Can you work these out from the model? Positions are in its coordinate system, mm. Coordinates: 2 decimals unless noted, no trailing zeros. Write item = value, one per line.
```python
from build123d import *

# Parameters (mm, degrees)
F1_DEPTH = 504


with BuildPart() as f1:
    # F0 (on Top) → F1 (new body)
    with BuildSketch(Plane.XY):
        Polygon((12, 4), (-12, 4), (-12, -4), (-1.9, -4), (-1.9, 2.8), (1.9, 2.8), (1.9, -4), (12, -4), align=None)
        with BuildLine():
            Line((-9.623275, -3.2), (-11.2, -3.2))
            Line((-11.2, -3.2), (-11.2, 3.2))
            Line((-11.2, 3.2), (-9.623275, 3.2))
            ThreePointArc((-9.623275, 3.2), (-9.422747, 2.985045), (-9.502111, 2.701993))
            Line((-9.502111, 2.701993), (-10.097086, 2.107018))
            ThreePointArc((-10.097086, 2.107018), (-10.312788, 1.783105), (-10.388512, 1.401382))
            Line((-10.388512, 1.401382), (-10.388512, 1.218503))
            ThreePointArc((-10.388512, 1.218503), (-10.25826, 1.031059), (-10.03716, 1.087764))
            ThreePointArc((-10.03716, 1.087764), (-8.786443, 1.659163), (-7.537162, 1.084629))
            ThreePointArc((-7.537162, 1.084629), (-7.316853, 1.031709), (-7.188512, 1.218431))
            Line((-7.188512, 1.218431), (-7.188512, 1.397588))
            ThreePointArc((-7.188512, 1.397588), (-7.264631, 1.780269), (-7.481401, 2.104691))
            Line((-7.481401, 2.104691), (-8.076376, 2.699666))
            ThreePointArc((-8.076376, 2.699666), (-8.154767, 2.986603), (-7.947546, 3.2))
            Line((-7.947546, 3.2), (-2.8, 3.2))
            Line((-2.8, 3.2), (-2.8, -3.2))
            Line((-2.8, -3.2), (-7.947546, -3.2))
            ThreePointArc((-7.947546, -3.2), (-8.154767, -2.986603), (-8.076376, -2.699666))
            Line((-8.076376, -2.699666), (-7.481401, -2.104691))
            ThreePointArc((-7.481401, -2.104691), (-7.264631, -1.780269), (-7.188512, -1.397588))
            Line((-7.188512, -1.397588), (-7.188512, -1.218431))
            ThreePointArc((-7.188512, -1.218431), (-7.316853, -1.031709), (-7.537162, -1.084629))
            ThreePointArc((-7.537162, -1.084629), (-8.786443, -1.659163), (-10.03716, -1.087764))
            ThreePointArc((-10.03716, -1.087764), (-10.25826, -1.031059), (-10.388512, -1.218503))
            Line((-10.388512, -1.218503), (-10.388512, -1.401382))
            ThreePointArc((-10.388512, -1.401382), (-10.312788, -1.783105), (-10.097086, -2.107018))
            Line((-10.097086, -2.107018), (-9.502111, -2.701993))
            ThreePointArc((-9.502111, -2.701993), (-9.422747, -2.985045), (-9.623275, -3.2))
        make_face(mode=Mode.SUBTRACT)
        with BuildLine():
            Line((7.188512, 1.397588), (7.188512, 1.218431))
            ThreePointArc((7.188512, 1.218431), (7.316853, 1.031709), (7.537162, 1.084629))
            ThreePointArc((7.537162, 1.084629), (8.786443, 1.659163), (10.03716, 1.087764))
            ThreePointArc((10.03716, 1.087764), (10.25826, 1.031059), (10.388512, 1.218503))
            Line((10.388512, 1.218503), (10.388512, 1.401382))
            ThreePointArc((10.388512, 1.401382), (10.312788, 1.783105), (10.097086, 2.107018))
            Line((10.097086, 2.107018), (9.502111, 2.701993))
            ThreePointArc((9.502111, 2.701993), (9.422747, 2.985045), (9.623275, 3.2))
            Line((9.623275, 3.2), (11.2, 3.2))
            Line((11.2, 3.2), (11.2, -3.2))
            Line((11.2, -3.2), (9.623275, -3.2))
            ThreePointArc((9.623275, -3.2), (9.422747, -2.985045), (9.502111, -2.701993))
            Line((9.502111, -2.701993), (10.097086, -2.107018))
            ThreePointArc((10.097086, -2.107018), (10.312788, -1.783105), (10.388512, -1.401382))
            Line((10.388512, -1.401382), (10.388512, -1.218503))
            ThreePointArc((10.388512, -1.218503), (10.25826, -1.031059), (10.03716, -1.087764))
            ThreePointArc((10.03716, -1.087764), (8.786443, -1.659163), (7.537162, -1.084629))
            ThreePointArc((7.537162, -1.084629), (7.316853, -1.031709), (7.188512, -1.218431))
            Line((7.188512, -1.218431), (7.188512, -1.397588))
            ThreePointArc((7.188512, -1.397588), (7.264631, -1.780269), (7.481401, -2.104691))
            Line((7.481401, -2.104691), (8.076376, -2.699666))
            ThreePointArc((8.076376, -2.699666), (8.154767, -2.986603), (7.947546, -3.2))
            Line((7.947546, -3.2), (2.8, -3.2))
            Line((2.8, -3.2), (2.8, 3.2))
            Line((2.8, 3.2), (7.947546, 3.2))
            ThreePointArc((7.947546, 3.2), (8.154767, 2.986603), (8.076376, 2.699666))
            Line((8.076376, 2.699666), (7.481401, 2.104691))
            ThreePointArc((7.481401, 2.104691), (7.264631, 1.780269), (7.188512, 1.397588))
        make_face(mode=Mode.SUBTRACT)
    extrude(amount=F1_DEPTH)


solid = f1.part
```
Item 1: I'm going to push flat-ended pins straight in: P1, Ø4, axis at x = -9, y = -3, coming from the -Z side; P2, Ø1, axis at x = -6.5, y = 0.5, coming from the -Z side; P3, Ø1.9, axis at x = 0.5, z = 177, coming from the -Y side. Where does each tip first touch, or does it pass through?
A:
P1 = 0
P2 = through
P3 = 2.8
Item 2: If I drill on probe 1 along X at (y, z) = (0.25, 326); probe 2 along Y at (x, z) = (8, 34.5); probe 3 along X at (y, z) = (-3, 266.5), over which ranges is the centre line in solid material (lowest first)?
A:
probe_1 = -12 to -11.2, -2.8 to -1.9, 1.9 to 2.8, 11.2 to 12
probe_2 = -4 to -3.18, -2.62 to -1.46, 1.46 to 2.62, 3.18 to 4
probe_3 = -12 to -11.2, -9.43 to -8.15, -2.8 to -1.9, 1.9 to 2.8, 8.15 to 9.43, 11.2 to 12
Item 3: I want a section at A-A, the plane z = 166.5. Give the number of separate pieces and of enclosed holes in the cut face, plus the area to 3 significant figures.
A:
separate_pieces = 1
enclosed_holes = 2
area = 74.8 mm2
